Autodesk Inventor part; units mm, degrees
ref_plane "Work Plane1" through (1.525, 0, 0) normal (0, 0, 1) x (1, 0, 0)
ref_plane "YZ Plane" through (0, 0, 0) normal (1, 0, 0) x (0, 1, 0)
ref_plane "XZ Plane" through (0, 0, 0) normal (0, 1, 0) x (-1, 0, 0)
sketch "Sketch1" plane through (0, 0, 0) normal (0, 0, 1) x (1, 0, 0)
  line L0 (0, 2.5) -> (0, 1.25)
  line L1 (1.3, 1.25) -> (6, 1.25)
  line L2 (6, 1.25) -> (6, 0)
  line L3 (6, 0) -> (-0.0011, 0)
  line L4 (-1.2013, 0) -> (7.2002, 0)
  line L5 (-0.0011, 0) -> (-0.0011, 2.5)
  line L6 (-0.0011, 2.5) -> (0, 2.5)
  line L7 (1.3, 1.25) -> (1.0238, 1.25)
  line L8 (1.0238, 1.25) -> (0, 1.25)
  line L9 (0, -0.5) -> (0, 3)
  dimension "d0" = 6
  dimension "d1" = 4.7
  dimension "d2" = 2.5
  dimension "d9" = 0.0011
  dimension "d10" = 5
  dimension "d13" = 0.2762
  dimension "d14" = 2.5
revolve "Body" add sketch "Sketch1" angle 360 about axis through (6, 0, 0) along (-1, 0, 0)
sketch "Sketch2" plane through (-0.0011, 0, 0) normal (-1, 0, 0) x (0, 0, 1)
  line L0 (0, 2.8868) -> (2.5, 1.4434)
  line L1 (2.5, 1.4434) -> (2.5, -1.4434)
  line L2 (2.5, -1.4434) -> (0, -2.8868)
  line L3 (0, -2.8868) -> (-2.5, -1.4434)
  line L4 (-2.5, -1.4434) -> (-2.5, 1.4434)
  line L5 (-2.5, 1.4434) -> (0, 2.8868)
  point P0 (0, 0)
  point P1 (0, 0)
  dimension "d11" = 5
extrude "Head" add sketch "Sketch2" along normal blind 5
sketch "Sketch4" plane through (0, 0, 0) normal (0, 0, 1) x (1, 0, 0)
  line L0 (-5.0011, 2.5) -> (-5.0011, 2.8868)
  line L1 (-5.0011, 2.8868) -> (-4.7778, 2.8868)
  line L2 (-4.7778, 2.8868) -> (-5.0011, 2.5)
  line L3 (-2.0399, 0) -> (0.3387, 0)
  line L4 (-0.0011, 2.8868) -> (-5.0011, 2.8868)
  line L5 (-5.0011, 1.4434) -> (-5.0011, 2.8868)
  line L6 (-0.0011, -2.8868) -> (-5.0011, -2.8868)
  line L7 (-0.0011, 2.1651) -> (-0.0011, 2.8868)
  line L8 (-0.0011, 2.8868) -> (-0.2244, 2.8868)
  dimension "d5" = 30
  dimension "d19" = 5
revolve "Chamfer1" cut sketch "Sketch4" angle 360 about axis through (-10, 0, 0) along (1, 0, 0)
thread "Thread"
chamfer "Chamfer2" distance 0.2761 distance2 0.2762 1 edges at (6, -1.25, 0) measured on face at (6, -0.3871, 0.3429)
ref_plane "Work Plane1" through (1.525, 0, 0) normal (0, 0, 1) x (1, 0, 0)
sketch "Sketch7" plane through (-5.0011, 0, 0) normal (-1, 0, 0) x (0, 0, 1)
  circle A0 centre (0, 0) radius 1.45
  point P0 (0, 0)
  dimension "d59" = 2.9
extrude "Extrusion5" cut sketch "Sketch7" against normal blind 4
equation "\"d11\" = SW"
equation "\"d15\" = GEL"
equation "\"d6\" = -0.5 * SPD + 0.5 * GD"
equation "\"d0\" = NLG"
equation "\"d1\" = GEL"
equation "\"d2\" = GD"
equation "\"d10\" = SD2"
equation "\"d14\" = BDM"
equation "\"d5\" = ANG1"
equation "\"d19\" = SW0"
equation "\"NLG\" = 6"
equation "\"GD\" = NND"
equation "\"BDM\" = NND"
equation "\"KOH\" = 1.7"
equation "\"GEL\" = 4.7"
equation "\"SW\" = 5"
equation "\"SW0\" = SW"
equation "\"SPD\" = NND - 1.2269 * PTC"
equation "\"SD2\" = SW"
equation "\"SD\" = 0.001"
equation "\"ANG1\" = 30deg"
equation "\"GAL\" = 0.61345 * PTC"
equation "\"GUL\" = 0.61345 * PTC"
equation "\"RR\" = 0.001"
equation "\"WFT\" = SD"
equation "\"GD1\" = THREADDIA - 1.2269 * PTC"
equation "\"THREADDIA\" = 2.5"
equation "\"SDH\" = SW"
equation "\"TOA\" = 30deg"
equation "\"FAWI\" = 45deg"
equation "\"PTC\" = 0.45"
equation "\"NND\" = 2.5"
equation "\"E0\" = 1.155 * SW"
properties part number "AS 1110 - M2.5 x 6" material "Steel, Mild"
Part model, mm, in its own coordinate system. A direction names the side the tool comes from. Coordinates: 2 decimals unless noted, no trailing zeros. Write each loop counter-clockwise with the first axis right and the second up, starting at its lowest first coordinate (ties: lowest second). Pieces come first, ordered by that corner, then holes.
Item 1: Mould opens along Y. For faces 4 (the face through (2.9, -0.27, -1.22)), 5 (the face through (-1.001, 0, 0)), 6 (the face through (-4.905, 1.338, 2.305)), 7 (the face through (-2.466, -2.175, -1.233)) say: released by +Y, released by -Y, zero draft, split by the parting line, or undercut.
Item 2: Probe line 1 (X direction, y = 0.8, z = 1.1); line 2 (X direction, y = -0.1, z = -0.15); line 3 (Z direction, x = -2, y = -0.85). List the from-to ranges inside material, lowest first.
Item 3: Slice it at B-B (x = 1.25). Write the cut outline in (y, z).
Item 4: Which spindle directions (+Z, -Z, +X, -X, +Y, -Y) get a long thin tool onto all of the face, cutting with end or side? Do faces 1 (the face through (-0.001, -1, -1)), 2 (the face through (-3.03, 0.06, -1.45)), 3 (the face through (-4.92, 1.31, -2.29)). Say none if no direction does.
Item 5: Pin check, flat tips, straight feed: pin 1 (1.7 mm diameter, centred on y = 0, z = 0, fed in from -X); pin 2 (2.5 mm diameter, centred on y = 0.5, z = 0, fed in from -X); pin 3 (1.5 mm diameter, centred on x = -3, z = 0.5, fed in from -Y). Stop position of each tip, or through.
Item 6: Slice it at A-A (x = -4). Write the cut outline in (y, z).
Results found:
1. face 4: split by the parting line
1. face 5: undercut
1. face 6: released by +Y
1. face 7: released by -Y
2. line 1: x = -1 to 0
2. line 2: x = -1 to 6
2. line 3: z = -2.5 to -1.17, 1.17 to 2.5
3. outline: circle Ø2.5 at (0, 0)
4. face 1: +X
4. face 2: -X
4. face 3: -Z, -X, +Y
5. pin 1: stops at x = -1
5. pin 2: stops at x = -5
5. pin 3: stops at y = -2.89
6. outline: (-2.89, 0) - (-1.44, -2.5) - (1.44, -2.5) - (2.89, 0) - (1.44, 2.5) - (-1.44, 2.5) - close; hole circle Ø2.9 at (0, 0)
